```python
from build123d import *

# Parameters (mm, degrees)
F1_DEPTH = 102
F2_R     = 6
F3_DEPTH = 50
F4_R     = 6
F5_DEPTH = 4


with BuildPart() as f1:
    # F0 (on Front) → F1 (new body)
    with BuildSketch(Plane.XZ):
        with BuildLine():
            Line((-41, 4), (0, 4))
            Line((0, 4), (41, 4))
            Line((41, 4), (42, 46))
            Line((42, 46), (41.5, 60))
            Line((41.5, 60), (20, 73))
            ThreePointArc((20, 73), (0, 59), (-20, 73))
            Line((-20, 73), (-41.5, 60))
            Line((-41.5, 60), (-42, 46))
            Line((-42, 46), (-41, 4))
        make_face()
    extrude(amount=-F1_DEPTH)

    # F2 (on face) → F3 (join)
    with BuildSketch(Plane(origin=(0, 102, 0), x_dir=(-1, 0, 0), z_dir=(0, 1, 0))):
        with Locations((0, 32)):
            Circle(F2_R)
    extrude(amount=F3_DEPTH)

    # F4 (on face) → F5 (join)
    with BuildSketch(Plane(origin=(0, 0, 4), x_dir=(1, 0, 0), z_dir=(0, 0, -1))):
        with Locations((29, -94)):
            Circle(F4_R)
        with Locations((-29, -94)):
            Circle(F4_R)
        with Locations((-29, -8)):
            Circle(F4_R)
        with Locations((29, -8)):
            Circle(F4_R)
    extrude(amount=F5_DEPTH)


solid = f1.part
```
The listing builds one solid part. Answer for the finished solid, in the listing's coordinates (mm). A direction names the side the tool comes from. Round coordinates to 2 decimals unless told otherwise and drop trailing zeros. Loops run counter-clockwise (first coordinate to the right, second up) from the corner with the lowest first, then second, coordinate; pieces in that order, holes last. Notation, with made-up numbers: (25, 75.25) - (61, 75.25) arc R18 ccw to (61, 83.25) - close; hole circle Ø11 at (-40, -26). An arc over 180 degrees is marked (long way). Use one line per item in the form item = value. Start each with the question number.
1. The part is cut by section A-A on z = 65. Determine the outline of the cut face in (x, y), then the cut area to 3 significant figures.
2. The part is cut by section C-C on x = 26. Determine the outline of the cut face in (y, z).
3. The part is cut by section D-D on y = 8. Determine the outline of the cut face in (x, z).
4. Consider line 1 (Y direction, x = 14, z = 18); line 2 (X direction, y = 79.5, z = 63.5); line 3 (X direction, y = 61, z = 43.5). Determine where each line is inside the solid, lowest interval first. Write a range as [from, to].
5. For a pull along Y with two mould halves and no side action, classify faces 1 (the face through (-1, 102, 39)), 2 (the face through (-33.42, 89.94, 2.03)), 3 (the face through (-30.6, 50.29, 66.59)) as pulls with the +Y half, pulls with the -Y half, needs draft (parallel to the pull), parting line crosses it, or undercut.
6. The part is cut by section B-B on y = 32.5. Determine the outline of the cut face in (x, z), then the cut area to 3 significant figures.
7. Given pin 1 Ø1.5 at (x, y) = (2.5, 25) entering from -Z; pin 2 Ø2 at (x, y) = (28.5, 94.5) entering from -Z; pin 3 Ø3 at (y, z) = (18, 56) entering from +X; pin 4 Ø6 at (x, z) = (-19, 33.5) entering from +Y, each flat-ended and moving along its own axis, determine where each tip first touches the part or whether it passes through.
8. A tool of negligible diameter and unlimited length cuts with its end or side. For faces 4 (the face through (1.301, 126.65, 26.143)), 5 (the face through (24.58, 89.94, 2.03)), 6 (the face through (0, 50, 59)), from which of +Z, -Z, +X, -X, +Y, -Y can it reach the whole face along a straight path? Write none if from no direction.
Geometry check:
q1.outline = (-33.23, 0) - (-14.81, 0) - (-14.81, 102) - (-33.23, 102) - close; (14.81, 0) - (33.23, 0) - (33.23, 102) - (14.81, 102) - close
q1.area = 3,760 mm^2
q2.outline = (0, 4) - (2.8, 4) - (2.8, 0) - (13.2, 0) - (13.2, 4) - (88.8, 4) - (88.8, 0) - (99.2, 0) - (99.2, 4) - (102, 4) - (102, 69.37) - (0, 69.37) - close
q3.outline = (-42, 46) - (-41, 4) - (-35, 4) - (-35, 0) - (-23, 0) - (-23, 4) - (23, 4) - (23, 0) - (35, 0) - (35, 4) - (41, 4) - (42, 46) - (41.5, 60) - (20, 73) arc R21.29 cw to (-20, 73) - (-41.5, 60) - close
q4.line_1 = [0, 102]
q4.line_2 = [-35.71, -13.09], [13.09, 35.71]
q4.line_3 = [-41.94, 41.94]
q5.face_1 = pulls with the +Y half
q5.face_2 = undercut
q5.face_3 = needs draft
q6.outline = (-42, 46) - (-41, 4) - (41, 4) - (42, 46) - (41.5, 60) - (20, 73) arc R21.29 cw to (-20, 73) - (-41.5, 60) - close
q6.area = 5,050 mm^2
q7.pin_1 = 4
q7.pin_2 = 0
q7.pin_3 = 41.7
q7.pin_4 = 102
q8.face_4 = +Y
q8.face_5 = -Z
q8.face_6 = +Z, +Y, -Y
